Job drawing, mm, ordinate dimensions from the low corner. One solid piece. Give positions to 0.01 mm unless a question says otherwise; leave off trailing zeros. Write each loop counter-clockwise with the first axis right and the second up, starting at its lowest first coordinate (ties: lowest second). Pieces come first, ordered by that corner, then holes. Notation, with made-up numbers: M 17.5,78.5 L 68.5,78.5 A30 ccw 68.5,112.5 Z; hole C 17.25,-30.75 d5. An arc over 180 degrees is marked long. Use CSV: the item, a comma, the result in double quotes. Start each with the question number.
Item 1: Pin check, flat tip, straight feed: pin 1 (8 mm diameter, centred on y = 11, z = 7, fed in from -X). Stop position of the tip, or through.
Item 2: Drill centre lines: line 1 (Z direction, x = 15, y = 12.5); line 2 (X direction, y = 9.25, z = 9.5); line 3 (Z direction, x = 24.5, y = 2). Where is each one in solid material? Low to high. Write a range as [from, to].
Item 3: Cut at A-A (x = 5). List the corners of the cut face in (y, z), then the cut area to 3 significant figures.
Item 4: Mould opens along Z. For the marked faces 1, 2 and 3 say: released by +Z, released by -Z, zero draft, split by the parting line, or undercut.
Item 5: Cut at B-B (z = 10). List the corners of the cut face in (x, y).
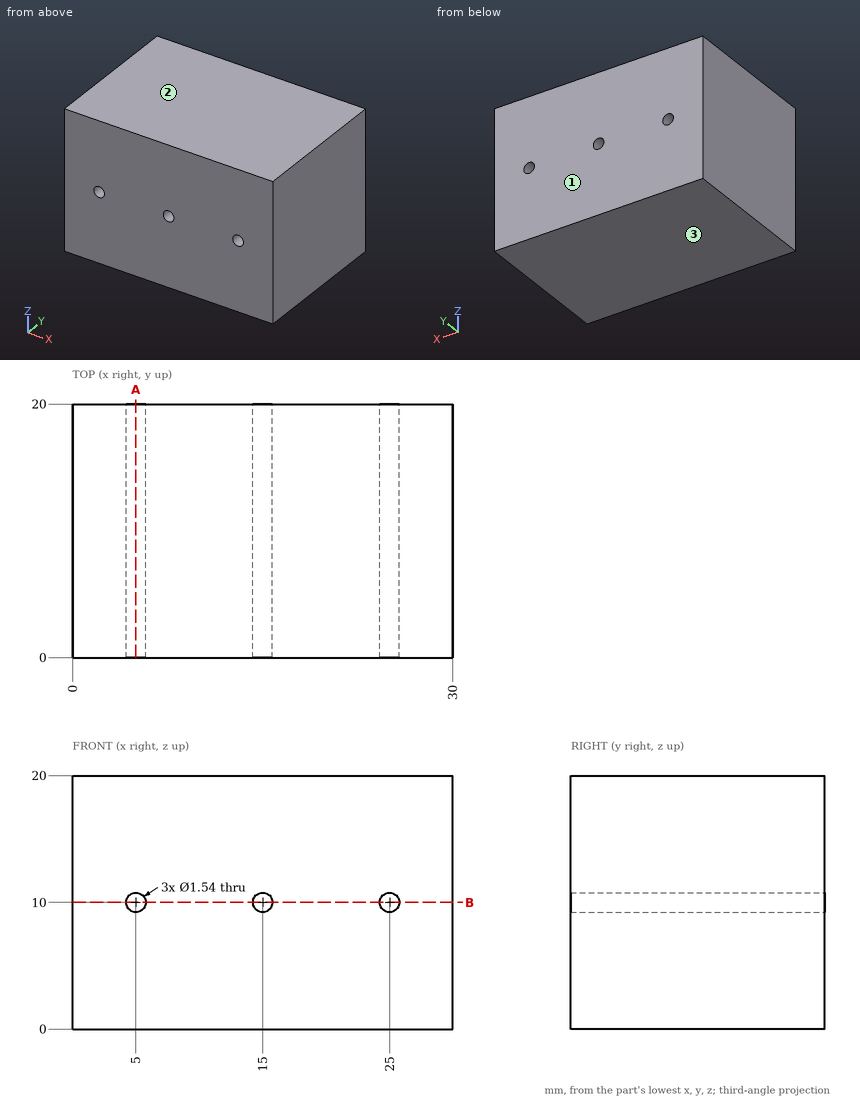
Worked answers:
1,pin 1,"stops at x = 0"
2,line 1,"z = [0, 9.23], [10.77, 20]"
2,line 2,"x = [0, 4.41], [5.59, 14.41], [15.59, 24.41], [25.59, 30]"
2,line 3,"z = [0, 9.41], [10.59, 20]"
3,outline,"M 0,0 L 20,0 L 20,9.23 L 0,9.23 Z; M 0,10.77 L 20,10.77 L 20,20 L 0,20 Z"
3,area,"369 mm^2"
4,face 1,"zero draft"
4,face 2,"released by +Z"
4,face 3,"released by -Z"
5,outline,"M 0,0 L 4.23,0 L 4.23,20 L 0,20 Z; M 5.77,0 L 14.23,0 L 14.23,20 L 5.77,20 Z; M 15.77,0 L 24.23,0 L 24.23,20 L 15.77,20 Z; M 25.77,0 L 30,0 L 30,20 L 25.77,20 Z"
